from build123d import *

# Parameters (mm, degrees)
SKETCH2_R           = 3.5
SKETCH2_R_2         = 1.5
BOSS_EXTRUDE1_DEPTH = 22
SKETCH3_W           = 1
SKETCH3_H           = 1
BOSS_EXTRUDE2_DEPTH = 1


with BuildPart() as part:
    # Sketch2 → Boss-Extrude1 (new body)
    with BuildSketch(Plane(origin=(0, 0, 0), x_dir=(1, 0, 0), z_dir=(0, 1, 0))):
        with Locations(Location((0, 0, 0), (0, 0, 270))):
            Circle(SKETCH2_R)
        with Locations(Location((0, 0, 0), (0, 0, 270))):
            Circle(SKETCH2_R_2, mode=Mode.SUBTRACT)
    extrude(amount=BOSS_EXTRUDE1_DEPTH)

    # Sketch3 → Boss-Extrude2 (add)
    with BuildSketch(Plane(origin=(0, 22, 0), x_dir=(1, 0, 0), z_dir=(0, 1, 0))):
        with Locations((0, 2.5)):
            Rectangle(SKETCH3_W, SKETCH3_H)
        with Locations((0, -2.5)):
            Rectangle(SKETCH3_W, SKETCH3_H)
    boss_extrude2 = extrude(amount=BOSS_EXTRUDE2_DEPTH)

    # Mirror1: Boss-Extrude2 across plane
    add(boss_extrude2.mirror(Plane.ZX.offset(11)))


solid = part.part
Design review of the part built by this model. Coordinates are the model's own, in mm. A direction names the side the tool comes from. Coordinates: 2 decimals unless noted, no trailing zeros. Write each loop counter-clockwise with the first axis right and the second up, starting at its lowest first coordinate (ties: lowest second). Pieces come first, ordered by that corner, then holes. Notation, with made-up numbers: (62.5, 63) -> (111.5, 63) arc R21 cw to (111.5, 98) -> close; hole circle Ø11 at (52, 8.25). An arc over 180 degrees is marked (long way). Write each question's results on one line, items separated by ' | '. Start each with the question number.
(1) Take a section at C-C on y = 13.5. Write out the cut boundary in (x, z), and give its area (3 significant figures).
(2) Take a section at D-D on x = -1.25. Write out the cut boundary in (y, z), and give its area (3 significant figures).
(3) Clearance check with flat-ended pins moving along their axes: P1, Ø0.8, axis at x = 0, y = 22.5, coming from the -Z side; P2, Ø0.5, axis at x = 0, y = -0.5, coming from the +Z side; P3, Ø0.8, axis at y = 22.5, z = -2.5, coming from the -X side; P4, Ø1.5, axis at x = 0, z = 0, coming from the -Y side. State where each tip first meets the part, or that it passes through.
(4) The part is to be moulded in two halves that separate along Z. For faces 5 (the face through (-3.417, 10.846, -0.759)), 6 (the face through (0, 22.5, -2)), 7 (the face through (0.5, -0.5, -2.5)), say which applies: pulls with the +Z half, pulls with the -Z half, needs draft (parallel to the pull), parting line crosses it, or undercut.
(5) Take a section at A-A on z = 0. Write out the cut boundary in (x, y), and give its area (3 significant figures).
(6) Take a section at B-B on x = 0. Write out the cut boundary in (y, z).
(7) For line 1 along X through (y, z) = (17.5, 0); line 2 along Y through (x, z) = (-1.5, -0.5); line 3 along Z through (x, y) = (1.25, 19.25), list the stretches that pass through material, from the lowest coordinate up. Write a range as from..to.
(8) Tool access review of faces 1 (the face through (0.5, 22.5, 2.5)), 2 (the face through (0, 22.5, 2)), 3 (the face through (0, -0.5, -2)), 4 (the face through (-0.5, -0.5, 2.5)): name each direction out of +Z, -Z, +X, -X, +Y, -Y from which nothing blocks a thin tool from reaching the whole face with its end or side.
Results found:
1) outline: circle Ø7 at (0, 0); hole circle Ø3 at (0, 0) | area: 31.4 mm2
2) outline: (0, -3.27) -> (22, -3.27) -> (22, -0.83) -> (0, -0.83) -> close; (0, 0.83) -> (22, 0.83) -> (22, 3.27) -> (0, 3.27) -> close | area: 107 mm2
3) P1: stops at z = -3 | P2: stops at z = 3 | P3: stops at x = -0.5 | P4: passes through
4) face 5: parting line crosses it | face 6: undercut | face 7: needs draft
5) outline: (-3.5, 0) -> (-1.5, 0) -> (-1.5, 22) -> (-3.5, 22) -> close; (1.5, 0) -> (3.5, 0) -> (3.5, 22) -> (1.5, 22) -> close | area: 88.0 mm2
6) outline: (-1, -3) -> (0, -3) -> (0, -3.5) -> (22, -3.5) -> (22, -3) -> (23, -3) -> (23, -2) -> (22, -2) -> (22, -1.5) -> (0, -1.5) -> (0, -2) -> (-1, -2) -> close; (-1, 2) -> (0, 2) -> (0, 1.5) -> (22, 1.5) -> (22, 2) -> (23, 2) -> (23, 3) -> (22, 3) -> (22, 3.5) -> (0, 3.5) -> (0, 3) -> (-1, 3) -> close
7) line 1: x = -3.5..-1.5, 1.5..3.5 | line 2: y = 0..22 | line 3: z = -3.27..-0.83, 0.83..3.27
8) face 1: +Z, -Z, +X, +Y | face 2: +X, -X, +Y | face 3: +X, -X, -Y | face 4: +Z, -Z, -X, -Y
